Build history of the part. All positions in model axes, mm. A direction names the side the tool comes from. Give positions to 0.01 mm unless a question says otherwise; leave off trailing zeros. Loops run counter-clockwise (first coordinate to the right, second up) from the corner with the lowest first, then second, coordinate; pieces in that order, holes last. Notation, with made-up numbers: (37, 80.5) -> (94, 80.5) arc R21 ccw to (94, 86.5) -> close; hole circle Ø2 at (-37.5, 53.25). An arc over 180 degrees is marked (long way). Answer as a JSON object with one key per item and string values. Group by question number.
from build123d import *

# Parameters (mm, degrees)
SKETCH1_W           = 20.32
SKETCH1_H           = 2.032
SKETCH1_R           = 4.445
BOSS_EXTRUDE1_DEPTH = 50.8
SKETCH2_R           = 2.54
CUT_EXTRUDE1_DEPTH  = 50.8
SKETCH1_3_R         = 4.445
CUT_EXTRUDE2_DEPTH  = 8.89
CUT_EXTRUDE3_START  = 20.32
SKETCH1_5_R         = 4.445
CUT_EXTRUDE3_DEPTH  = 8.89
SKETCH3_R           = 2.54
CUT_EXTRUDE4_DEPTH  = 60.369104181
CUT_EXTRUDE5_START  = 41.91
SKETCH1_6_R         = 4.445
CUT_EXTRUDE5_DEPTH  = 8.89


with BuildPart() as part:
    # Sketch1 → Boss-Extrude1 (new body)
    with BuildSketch(Plane(origin=(0, 0, 0), x_dir=(1, 0, 0), z_dir=(0, 1, 0))):
        with Locations((10.16, 1.016)):
            Rectangle(SKETCH1_W, SKETCH1_H)
        with BuildLine():
            Line((21.032326163, 2.032), (20.32, 2.032))
            Line((20.32, 2.032), (20.32, 0))
            Line((20.32, 0), (21.995191819, 0))
            ThreePointArc((21.995191819, 0), (21.383144864, 0.954108338), (21.032326163, 2.032))
        make_face()
        with Locations((25.4, 2.8575)):
            Circle(SKETCH1_R)
    extrude(amount=BOSS_EXTRUDE1_DEPTH)

    # Sketch2 → Cut-Extrude1 (cut)
    with BuildSketch(Plane(origin=(0, 0, -2.032), x_dir=(-1, 0, 0), z_dir=(0, 0, -1))):
        with Locations((-7.62, 43.18)):
            Circle(SKETCH2_R)
        with Locations((-7.62, 7.62)):
            Circle(SKETCH2_R)
    extrude(amount=-CUT_EXTRUDE1_DEPTH, mode=Mode.SUBTRACT)

    # Sketch1_3 → Cut-Extrude2 (cut)
    with BuildSketch(Plane(origin=(0, 0, 0), x_dir=(1, 0, 0), z_dir=(0, 1, 0))):
        with BuildLine():
            Line((21.032326163, 2.032), (20.32, 2.032))
            Line((20.32, 2.032), (20.32, 0))
            Line((20.32, 0), (21.995191819, 0))
            ThreePointArc((21.995191819, 0), (21.383144864, 0.954108338), (21.032326163, 2.032))
        make_face()
        with Locations((25.4, 2.8575)):
            Circle(SKETCH1_3_R)
    extrude(amount=CUT_EXTRUDE2_DEPTH, mode=Mode.SUBTRACT)

    # Sketch1_5 → Cut-Extrude3 (cut)
    with BuildSketch(Plane(origin=(0, 0, 0), x_dir=(1, 0, 0), z_dir=(0, 1, 0)).offset(CUT_EXTRUDE3_START)):
        with Locations((25.4, 2.8575)):
            Circle(SKETCH1_5_R)
        with BuildLine():
            Line((21.032326163, 2.032), (20.32, 2.032))
            Line((20.32, 2.032), (20.32, 0))
            Line((20.32, 0), (21.995191819, 0))
            ThreePointArc((21.995191819, 0), (21.383144864, 0.954108338), (21.032326163, 2.032))
        make_face()
    extrude(amount=CUT_EXTRUDE3_DEPTH, mode=Mode.SUBTRACT)

    # Sketch3 → Cut-Extrude4 (cut, through all)
    with BuildSketch(Plane(origin=(0, 50.8, 0), x_dir=(1, 0, 0), z_dir=(0, 1, 0))):
        with Locations(Location((25.4, 2.8575, 0), (0, 0, 270))):
            Circle(SKETCH3_R)
    extrude(amount=-CUT_EXTRUDE4_DEPTH, mode=Mode.SUBTRACT)

    # Sketch1_6 → Cut-Extrude5 (cut)
    with BuildSketch(Plane(origin=(0, 0, 0), x_dir=(1, 0, 0), z_dir=(0, 1, 0)).offset(CUT_EXTRUDE5_START)):
        with Locations((25.4, 2.8575)):
            Circle(SKETCH1_6_R)
        with BuildLine():
            Line((21.032326163, 2.032), (20.32, 2.032))
            Line((20.32, 2.032), (20.32, 0))
            Line((20.32, 0), (21.995191819, 0))
            ThreePointArc((21.995191819, 0), (21.383144864, 0.954108338), (21.032326163, 2.032))
        make_face()
    extrude(amount=CUT_EXTRUDE5_DEPTH, mode=Mode.SUBTRACT)


solid = part.part
(1) Probe line 1 along Y through (x, z) = (7.62, -1.25); line 2 along Y through (x, z) = (28, -3.5); line 3 along Z through (x, y) = (5.25, 48.5). List the from-to ranges inside material, lowest first. Write a range as [from, to].
(2) Saw through at A-A on x = 7.62. List the corners of the cut face in (y, z).
(3) 3-axis set-ups, long thin cutter, end or side, ignore diameter. For faces 1 (the flat face through (28.2, 20.32, -2.9)), 2 (the flat face through (28.2, 8.89, -2.9)), 3 (the flat face through (20.32, 46, -1)), 4 (the cylindrical face through (27.92, 14.69, -3.19)): which of +Z, -Z, +X, -X, +Y, -Y reach the whole face in a straight line?
(4) Pin check, flat tips, straight feed: pin 1 (17.5 mm diameter, centred on x = 6.5, y = 17, fed in from +Z); pin 2 (6.5 mm diameter, centred on x = 5.5, y = 23, fed in from -Z); pin 3 (0.6 mm diameter, centred on y = 47, z = -0.5, fed in from +X); pin 4 (1 mm diameter, centred on y = 6.5, z = -5, fed in from +X). Stop position of each tip, or through.
(5) Saw through at C-C on x = 25.4. List the corners of the cut face in (y, z), plus the area to 3 significant figures.
(6) Pull direction Z, two halves, no side cores. Call faces 5 (the cylindrical face through (27.92, 35.65, -3.19)), 6 (the flat face through (11, 25, 0)), 7 (the cylindrical face through (7.95, 45.7, -1.03)): pulls with the +Z half, pulls with the -Z half, needs draft (parallel to the pull), parting line crosses it, or undercut.
(7) Saw through at D-D on y = 43.18. List the corners of the cut face in (x, z), plus the area to 3 significant figures.
(8) Saw through at B-B on z = -1. List the corners of the cut face in (x, y).
Calculated:
{
 "1": {"line 1": "y = [0, 5.08], [10.16, 40.64], [45.72, 50.8]", "line 2": "y = [8.89, 20.32], [29.21, 41.91]", "line 3": "z = [-2.03, 0]"},
 "2": {"outline": "(0, -2.03) -> (5.08, -2.03) -> (5.08, 0) -> (0, 0) -> close; (10.16, -2.03) -> (40.64, -2.03) -> (40.64, 0) -> (10.16, 0) -> close; (45.72, -2.03) -> (50.8, -2.03) -> (50.8, 0) -> (45.72, 0) -> close"},
 "3": {"face 1": "+Z, -Z, +X", "face 2": "+Z, -Z, +X, -Y", "face 3": "+Z, -Z, +X, +Y", "face 4": "+Y, -Y"},
 "4": {"pin 1": "stops at z = 0", "pin 2": "stops at z = -2.03", "pin 3": "stops at x = 20.32", "pin 4": "passes through"},
 "5": {"outline": "(8.89, -7.3) -> (20.32, -7.3) -> (20.32, -5.4) -> (8.89, -5.4) -> close; (8.89, -0.32) -> (20.32, -0.32) -> (20.32, 1.59) -> (8.89, 1.59) -> close; (29.21, -7.3) -> (41.91, -7.3) -> (41.91, -5.4) -> (29.21, -5.4) -> close; (29.21, -0.32) -> (41.91, -0.32) -> (41.91, 1.59) -> (29.21, 1.59) -> close", "area": "91.9 mm^2"},
 "6": {"face 5": "undercut", "face 6": "pulls with the +Z half", "face 7": "needs draft"},
 "7": {"outline": "(0, -2.03) -> (5.08, -2.03) -> (5.08, 0) -> (0, 0) -> close; (10.16, -2.03) -> (20.32, -2.03) -> (20.32, 0) -> (10.16, 0) -> close", "area": "31.0 mm^2"},
 "8": {"outline": "(0, 0) -> (20.32, 0) -> (20.32, 8.89) -> (23.67, 8.89) -> (23.67, 20.32) -> (20.32, 20.32) -> (20.32, 29.21) -> (23.67, 29.21) -> (23.67, 41.91) -> (20.32, 41.91) -> (20.32, 50.8) -> (0, 50.8) -> close; (27.13, 8.89) -> (29.44, 8.89) -> (29.44, 20.32) -> (27.13, 20.32) -> close; (27.13, 29.21) -> (29.44, 29.21) -> (29.44, 41.91) -> (27.13, 41.91) -> close; hole circle Ø5.08 at (7.62, 7.62); hole circle Ø5.08 at (7.62, 43.18)"}
}
